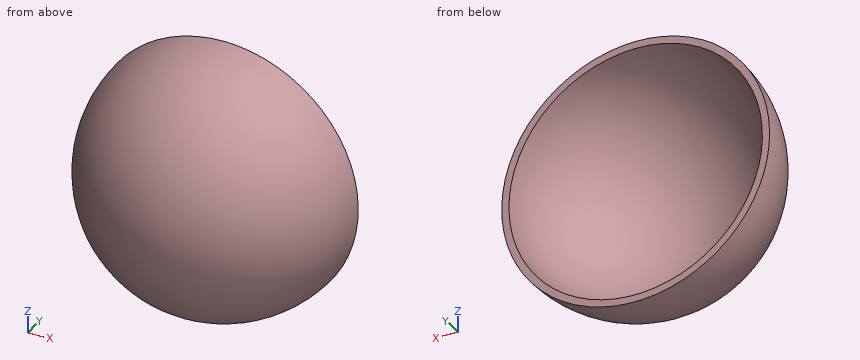
```python
from build123d import *

# Parameters (mm, degrees)
CROQUIS2_W            = 10
CROQUIS2_H            = 14
REDONDEO1_R           = 1
CROQUIS3_R            = 29.845650159
CORTAR_EXTRUIR1_DEPTH = 30


with BuildPart() as part:
    # Croquis1 → Revolución3 (revolve)
    with BuildSketch(Plane(origin=(0, 0, 0), x_dir=(0, 0, -1), z_dir=(1, 0, 0))):
        with BuildLine():
            Line((-0.5, 27.995535358), (-0.5, 26.495282599))
            Line((-0.5, 26.495282599), (-0.5, 24.9949995))
            ThreePointArc((-0.5, 24.9949995), (-10.791516482, 22.5509018), (-19.151111078, 16.069690242))
            Line((-19.151111078, 16.069690242), (-20.300177743, 17.033871657))
            ThreePointArc((-20.300177743, 17.033871657), (-24.017156356, -11.199383936), (0, -26.5))
            Line((0, -26.5), (0, -28))
            ThreePointArc((0, -28), (-27.998883817, -0.250009966), (-0.5, 27.995535358))
        make_face()
    revolve(axis=Axis((0, 29, 0), (0, -1, 0)))

    # Croquis2 → Cortar-Revolución2 (revolve, cut)
    with BuildSketch(Plane(origin=(0, 0, 0), x_dir=(0, 0, -1), z_dir=(1, 0, 0))):
        with Locations((-5, 23)):
            Rectangle(CROQUIS2_W, CROQUIS2_H)
    revolve(axis=Axis((0, 0, 0), (0, 1, 0)), mode=Mode.SUBTRACT)

    # Redondeo1
    redondeo1_edges = [part.edges().sort_by_distance(p)[0] for p in [
        (0, 22.912878475, -10),
        (0, 26.153393661, -10),
        (0, 16.069690242, -19.151111078),
    ]]
    fillet(redondeo1_edges, radius=REDONDEO1_R)

    # Croquis3 → Cortar-Extruir1 (cut)
    with BuildSketch(Plane(origin=(0, 0, 0), x_dir=(1, 0, 0), z_dir=(0, 1, 0))):
        Circle(CROQUIS3_R)
    extrude(amount=CORTAR_EXTRUIR1_DEPTH, mode=Mode.SUBTRACT)


solid = part.part
```
Could you check a few things on this model? Use its own coordinates, in mm. Coordinates: 2 decimals unless noted, no trailing zeros. Order: outer loops, then holes, each group sorted by start corner. A loop starts at its lowest first (then second) coordinate and runs counter-clockwise, first axis right, second up. Notation, with made-up numbers: M -35.5,-17.75 L -22.5,-17.75 A21 cw -22.5,6.25 Z; hole C 2.5,77.5 d4. An arc over 180 degrees is marked long. Use one line per item in the form item = value. Start each with the question number.
1. Suppose I cut it at C-C on z = -9. Write out the boundary of the cut face in (x, y).
2. Suppose I cut it at A-A on y = -10.75. Write out the boundary of the cut face in (x, z).
3. Please list where these lines run through material, in increasing order: line 1 (X direction, y = -21.5, z = -2); line 2 (Z direction, x = -18.5, y = -17.25); line 3 (Z direction, x = 0, y = -9.75).
4. For pin 1 (6 mm diameter, centred on y = -19, z = 13, fed in from -X); pin 2 (5 mm diameter, centred on x = -18.5, y = -20.5, fed in from -Z); pin 3 (2 mm diameter, centred on x = -10, z = -10, fed in from +Y), each with a flat end and sliding along its axis, tell me the tip position at first contact or that it passes through.
5. Suppose I cut it at B-B on x = 16.5. Write out the boundary of the cut face in (y, z).
Geometry says:
q1.outline = M -26.51,0 A26.51 ccw 26.51,0 L 24.92,0 A24.92 cw -24.92,0 Z
q2.outline = C 0,0 d51.71; hole C 0,0 d48.44
q3.line_1 = -17.83 to -15.36, 15.36 to 17.83
q3.line_2 = -12.01 to -7.9, 7.9 to 12.01
q3.line_3 = -26.25 to -24.64, 24.64 to 26.25
q4.pin_1 = -19.57
q4.pin_2 = -12.38
q4.pin_3 = -21.75
q5.outline = M 0,-22.62 L 0,-20.74 A20.74 cw 0,20.74 L 0,22.62 A22.62 ccw Z
